from build123d import *

# Parameters (mm, degrees)
SKETCH1_W           = 22.5
SKETCH1_H           = 11.8
BOSS_EXTRUDE1_DEPTH = 22.7
BOSS_EXTRUDE2_START = 15.9
BOSS_EXTRUDE2_DEPTH = 2.5
BOSS_EXTRUDE3_DEPTH = 4
SKETCH4_R           = 2.3
SKETCH4_R_2         = 0.85
BOSS_EXTRUDE4_DEPTH = 3.2
SKETCH5_W           = 3.6
SKETCH5_H           = 1.2
BOSS_EXTRUDE5_DEPTH = 1


with BuildPart() as part:
    # Sketch1 → Boss-Extrude1 (new body)
    with BuildSketch(Plane(origin=(0, 0, 0), x_dir=(1, 0, 0), z_dir=(0, 1, 0))):
        Rectangle(SKETCH1_W, SKETCH1_H)
    extrude(amount=BOSS_EXTRUDE1_DEPTH)

    # Sketch2 → Boss-Extrude2 (add)
    with BuildSketch(Plane(origin=(0, 0, 0), x_dir=(1, 0, 0), z_dir=(0, 1, 0)).offset(BOSS_EXTRUDE2_START)):
        with BuildLine():
            Line((15.95, 5.9), (11.25, 5.9))
            Line((11.25, 5.9), (11.25, -5.9))
            Line((11.25, -5.9), (15.95, -5.9))
            Line((15.95, -5.9), (15.95, -0.65))
            Line((15.95, -0.65), (14.409934208, -0.65))
            ThreePointArc((14.409934208, -0.65), (12.65, 0), (14.409934208, 0.65))
            Line((14.409934208, 0.65), (15.95, 0.65))
            Line((15.95, 0.65), (15.95, 5.9))
        make_face()
    boss_extrude2 = extrude(amount=BOSS_EXTRUDE2_DEPTH)

    # Mirror1: Boss-Extrude2 across plane
    add(boss_extrude2.mirror(Plane(origin=(0, 0, 0), x_dir=(0, 0, 1), z_dir=(1, 0, 0))))

    # Sketch3 → Boss-Extrude3 (add)
    with BuildSketch(Plane(origin=(0, 22.7, 0), x_dir=(1, 0, 0), z_dir=(0, 1, 0))):
        with BuildLine():
            ThreePointArc((-0.005844314, 2.5), (-11.25, 0), (-0.005844314, -2.5))
            Line((-0.005844314, -2.5), (0.95, -2.5))
            ThreePointArc((0.95, -2.5), (3.45, 0), (0.95, 2.5))
            Line((0.95, 2.5), (-0.005844314, 2.5))
        make_face()
    extrude(amount=BOSS_EXTRUDE3_DEPTH)

    # Sketch4 → Boss-Extrude4 (add)
    with BuildSketch(Plane(origin=(0, 26.7, 0), x_dir=(1, 0, 0), z_dir=(0, 1, 0))):
        with Locations((-5.35, 0)):
            Circle(SKETCH4_R)
        with Locations((-5.35, 0)):
            Circle(SKETCH4_R_2, mode=Mode.SUBTRACT)
    extrude(amount=BOSS_EXTRUDE4_DEPTH)

    # Sketch5 → Boss-Extrude5 (add)
    with BuildSketch(Plane(origin=(11.25, 0, 0), x_dir=(0, 0, -1), z_dir=(1, 0, 0))):
        with Locations((0, 5.1)):
            Rectangle(SKETCH5_W, SKETCH5_H)
    extrude(amount=BOSS_EXTRUDE5_DEPTH)


solid = part.part
Geometry: final body of the model. Coordinates: model frame, mm. A direction names the side the tool comes from. Give positions to 0.01 mm unless a question says otherwise; leave off trailing zeros. Loops run counter-clockwise (first coordinate to the right, second up) from the corner with the lowest first, then second, coordinate; pieces in that order, holes last. Notation, with made-up numbers: (72, -30.5) -> (98, -30.5) arc R10 cw to (98, -16.5) -> close; hole circle Ø4 at (-35.75, -29). An arc over 180 degrees is marked (long way). Put each result on its own line as item: value.
1. Cut plane D-D (y = 28). Return the cut outline in (x, z), plus the area to 3 significant figures.
Taken from the geometry:
outline: circle Ø4.6 at (-5.35, 0); hole circle Ø1.7 at (-5.35, 0)
area: 14.3 mm2
2. Cut plane C-C (z = -3.25). Return the cut outline in (x, y), plus the area to 3 significant figures.
Taken from the geometry:
outline: (-15.95, 15.9) -> (-11.25, 15.9) -> (-11.25, 0) -> (11.25, 0) -> (11.25, 15.9) -> (15.95, 15.9) -> (15.95, 18.4) -> (11.25, 18.4) -> (11.25, 22.7) -> (-0.43, 22.7) -> (-0.43, 26.7) -> (-10.27, 26.7) -> (-10.27, 22.7) -> (-11.25, 22.7) -> (-11.25, 18.4) -> (-15.95, 18.4) -> close
area: 574 mm2
3. Cut plane A-A (x = 13.65). Return the cut outline in (y, z), plus the area to 3 significant figures.
Taken from the geometry:
outline: (15.9, -5.9) -> (18.4, -5.9) -> (18.4, -1) -> (15.9, -1) -> close; (15.9, 1) -> (18.4, 1) -> (18.4, 5.9) -> (15.9, 5.9) -> close
area: 24.5 mm2
4. Ray query, line 1 along X through (y, z) = (28.1, 0); line 2 along Z through (x, y) = (13.65, 17.05); line 3 along Y through (x, z) = (14, 4.75). Return the intervals inside material, ascending. Write a range as [from, to].
Taken from the geometry:
line 1: x = [-7.65, -6.2], [-4.5, -3.05]
line 2: z = [-5.9, -1], [1, 5.9]
line 3: y = [15.9, 18.4]
5. Set-up query: faces 5 (the flat face through (5, 22.7, 0)), 6 (the flat face through (-10, 22.7, -4)), 7 (the flat face through (-2, 26.7, 0)). Return all of +Z, -Z, +X, -X, +Y, -Y with unobstructed straight access to the full face (end or side cutting, diameter ignored); none if empty.
Taken from the geometry:
face 5: +X, +Y
face 6: -Z, -X, +Y
face 7: +Y
6. Pull-direction query (X, two-part tool) for faces 1 (the cylindrical face through (12.65, 17.13, 0.03)), 2 (the flat face through (12, 5.7, 0)), 3 (the flat face through (-11.25, 8, 0)), 4 (the cylindrical face through (-12.65, 17.13, 0.03)); classes: released by +X, released by -X, zero draft, split by the parting line, or undercut.
Taken from the geometry:
face 1: undercut
face 2: zero draft
face 3: released by -X
face 4: undercut
7. Pin query (flat end, axial travel): P1, Ø0.8, axis at x = 12, z = -0.5, coming from the -Y side; P2, Ø2.5, axis at x = -13.5, z = 3, coming from the +Y side; P3, Ø1.5, axis at y = 4.5, z = -3.5, coming from the -X side. Return the tip coordinate at first contact, or that it passes through.
Taken from the geometry:
P1: stops at y = 4.5
P2: stops at y = 18.4
P3: stops at x = -11.25
8. Cut plane B-B (y = 18). Return the cut outline in (x, z).
Taken from the geometry:
outline: (-15.95, -5.9) -> (15.95, -5.9) -> (15.95, -0.65) -> (14.41, -0.65) arc R1 cw (long way) to (14.41, 0.65) -> (15.95, 0.65) -> (15.95, 5.9) -> (-15.95, 5.9) -> (-15.95, 0.65) -> (-14.41, 0.65) arc R1 cw (long way) to (-14.41, -0.65) -> (-15.95, -0.65) -> close
